Design review of the part shown in the three views and the two pictorial views. Dimensions are in mm from the part's minimum x, y and z. Coordinates: 2 decimals unless noted, no trailing zeros. Order: outer loops, then holes, each group sorted by start corner. A loop starts at its lowest first (then second) coordinate and runs counter-clockwise, first axis right, second up. Notation, with made-up numbers: (53, 8) -> (65, 8) arc R16 ccw to (65, 13) -> close; hole circle Ø1 at (88.5, -31). An arc over 180 degrees is marked (long way). Write item = value, one per line. Start each with the question number.
1) Insertion check: pin 1 Ø0.8 at (y, z) = (2, 10.5) entering from +X; pin 2 Ø1.5 at (x, y) = (7.5, 2) entering from -Z; pin 3 Ø2.5 at (x, z) = (24.5, 1.5) entering from +Y. Each pin has a flat end and moves straight along its axis. Give the tip position at first contact, or say it passes through.
2) Consider section D-D on x = 14.75. Give the boundary of the cut face in (y, z).
3) Consider section C-C on z = 12.75. Give the boundary of the cut face in (x, y).
4) Consider section A-A on z = 24.5. Give the boundary of the cut face in (x, y), and give its area (4 significant figures).
5) Consider section B-B on x = 24.5. Give the boundary of the cut face in (y, z), and give its area (3 significant figures).
6) Wall thickness on probe 1 along Z at (x, y) = (1.5, 0.55); probe 2 along Z at (x, y) = (19.75, 1.9); probe 3 along X at (y, z) = (1.6, 25.25): over which ranges is each line inside the solid? List them lowest first. Write a range as [from, to].
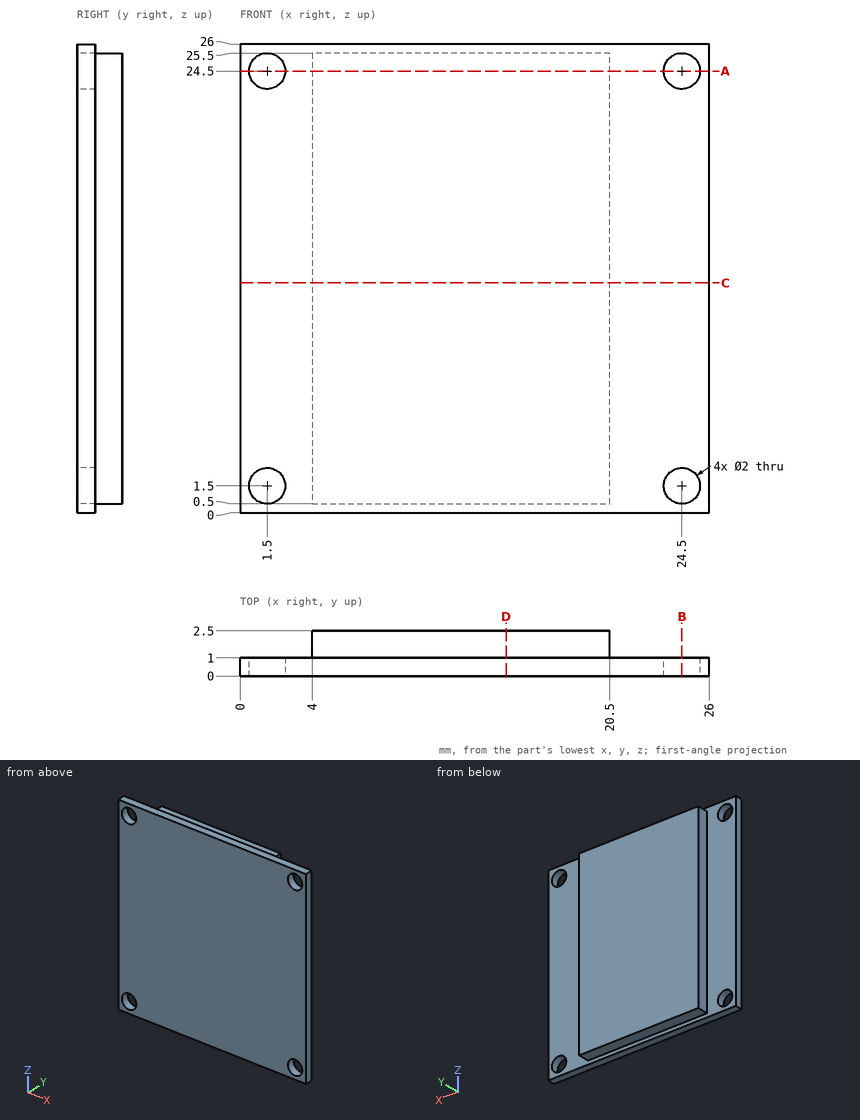
Answer sheet:
q1.pin_1 = 20.5
q1.pin_2 = 0.5
q1.pin_3 = 1
q2.outline = (0, 0) -> (1, 0) -> (1, 0.5) -> (2.5, 0.5) -> (2.5, 25.5) -> (1, 25.5) -> (1, 26) -> (0, 26) -> close
q3.outline = (0, 0) -> (26, 0) -> (26, 1) -> (20.5, 1) -> (20.5, 2.5) -> (4, 2.5) -> (4, 1) -> (0, 1) -> close
q4.outline = (0, 0) -> (0.5, 0) -> (0.5, 1) -> (0, 1) -> close; (2.5, 0) -> (23.5, 0) -> (23.5, 1) -> (20.5, 1) -> (20.5, 2.5) -> (4, 2.5) -> (4, 1) -> (2.5, 1) -> close; (25.5, 0) -> (26, 0) -> (26, 1) -> (25.5, 1) -> close
q4.area = 46.75 mm2
q5.outline = (0, 0) -> (1, 0) -> (1, 0.5) -> (0, 0.5) -> close; (0, 2.5) -> (1, 2.5) -> (1, 23.5) -> (0, 23.5) -> close; (0, 25.5) -> (1, 25.5) -> (1, 26) -> (0, 26) -> close
q5.area = 22.0 mm2
q6.probe_1 = [0, 0.5], [2.5, 23.5], [25.5, 26]
q6.probe_2 = [0.5, 25.5]
q6.probe_3 = [4, 20.5]
